The listing builds one solid part. Answer for the finished solid, in the listing's coordinates (mm). A direction names the side the tool comes from. Give positions to 0.01 mm unless a question says otherwise; leave off trailing zeros. Write each loop counter-clockwise with the first axis right and the second up, starting at its lowest first coordinate (ties: lowest second). Pieces come first, ordered by that corner, then holes. Notation, with made-up numbers: (42, -19.75) -> (65, -19.75) arc R28 ccw to (65, 19.25) -> close; hole circle Ø7 at (16, -37). An arc over 180 degrees is marked (long way). Put each result on its own line as item: value. Start each with the question number.
1) Find the intervals of material crossed by line 1 along X through (y, z) = (-0.8, 0); line 2 along Z through (x, y) = (0, 4.5), in increasing order. Write a range as from..to.
2) A cutting plane is placed at B-B (y = -0.5). Write down the section's boundary in (x, z).
3) For a pull along X with two mould halves and no side action, classify faces 1 (the cylindrical face through (-13.887, 1.577, 10.648)), 2 (the flat face through (0, -1.5, 0)), 3 (the flat face through (13, 3, -3.75)) as released by +X, released by -X, zero draft, split by the parting line, or undercut.
4) A cutting plane is placed at C-C (x = 0). Write down the section's boundary in (y, z).
5) A cutting plane is placed at A-A (z = 0). Write down the section's boundary in (x, y).
6) A cutting plane is placed at D-D (y = -2.75). Write down the section's boundary in (x, z), then the cut area to 3 significant figures.
7) Flat-ended cylindrical pins translate along their axes: pin 1 Ø2 at (x, y) = (12.5, 4.5) entering from -Z; pin 2 Ø2 at (x, y) = (13, 2) entering from +Z; pin 3 Ø1 at (y, z) = (-1.5, 13.5) entering from +X. Find the tip coordinate at first contact, or state that the pin passes through.
8) For faces 4 (the flat face through (14, 3, 3.75)), 5 (the flat face through (3, 0, 0)), 6 (the flat face through (0, -4, 0)), determine the directions among +Z, -Z, +X, -X, +Y, -Y from which every point of the face is accessible in a straight line to the end or side of a thin tool.
from build123d import *

# Parameters (mm, degrees)
SKETCH2_R           = 17.5
BOSS_EXTRUDE1_DEPTH = 4
BOSS_EXTRUDE2_DEPTH = 7
SKETCH2_4_R         = 1.2
CUT_EXTRUDE1_DEPTH  = 1.5


with BuildPart() as part:
    # Sketch2 → Boss-Extrude1 (new body)
    with BuildSketch(Plane(origin=(0, 0, 0), x_dir=(1, 0, 0), z_dir=(0, 1, 0))):
        Circle(SKETCH2_R)
    extrude(amount=-BOSS_EXTRUDE1_DEPTH)

    # Sketch2_3 → Boss-Extrude2 (add)
    with BuildSketch(Plane(origin=(0, 0, 0), x_dir=(1, 0, 0), z_dir=(0, 1, 0))):
        with BuildLine():
            Line((17.093492914, -3.75), (9.807522623, -3.75))
            ThreePointArc((9.807522623, -3.75), (-10.5, 0), (9.807522623, 3.75))
            Line((9.807522623, 3.75), (17.093492914, 3.75))
            ThreePointArc((17.093492914, 3.75), (-17.5, 0), (17.093492914, -3.75))
        make_face()
    extrude(amount=BOSS_EXTRUDE2_DEPTH)

    # Sketch2_4 → Cut-Extrude1 (cut)
    with BuildSketch(Plane(origin=(0, 0, 0), x_dir=(1, 0, 0), z_dir=(0, 1, 0))):
        Circle(SKETCH2_4_R)
    extrude(amount=-CUT_EXTRUDE1_DEPTH, mode=Mode.SUBTRACT)


solid = part.part
Reply:
1. line 1: x = -17.5..-1.2, 1.2..17.5
1. line 2: z = -17.5..-10.5, 10.5..17.5
2. outline: circle Ø35 at (0, 0); hole circle Ø2.4 at (0, 0)
3. face 1: split by the parting line
3. face 2: undercut
3. face 3: zero draft
4. outline: (-4, -17.5) -> (7, -17.5) -> (7, -10.5) -> (0, -10.5) -> (0, -1.2) -> (-1.5, -1.2) -> (-1.5, 1.2) -> (0, 1.2) -> (0, 10.5) -> (7, 10.5) -> (7, 17.5) -> (-4, 17.5) -> close
5. outline: (-17.5, -4) -> (17.5, -4) -> (17.5, 0) -> (1.2, 0) -> (1.2, -1.5) -> (-1.2, -1.5) -> (-1.2, 0) -> (-10.5, 0) -> (-10.5, 7) -> (-17.5, 7) -> close
6. outline: circle Ø35 at (0, 0)
6. area: 962 mm2
7. pin 1: stops at z = -13.19
7. pin 2: stops at z = 12.74
7. pin 3: stops at x = 11.72
8. face 4: +X, +Y
8. face 5: +Y
8. face 6: +Z, -Z, +X, -X, -Y
